Build history of the part. All positions in model axes, mm. Face numbers are marked on the shaded views. A direction names the side the tool comes from. Give positions to 0.01 mm unless a question says otherwise; leave off trailing zeros. Order: outer loops, then holes, each group sorted by start corner. A loop starts at its lowest first (then second) coordinate and runs counter-clockwise, first axis right, second up. Notation, with made-up numbers: (12.5, 2.5) -> (26.5, 2.5) arc R29 ccw to (26.5, 39.5) -> close; hole circle Ø2 at (12, 46.5). An arc over 180 degrees is marked (long way). One line per question, with ' | ' between items. Start each with the question number.
(1) Pull direction Z, two halves, no side cores. Call the marked faces 1, 2, 3 and 4: +Z half, -Z half, draft (parallel to the pull), parting line (faces both ways), or undercut.
(2) Cut at A-A (x = -23.95). Give the cut face in (y, z).
(3) Cut at C-C (y = -3). Give the cut face in (x, z), then the cut area to 3 significant figures.
(4) Cut at B-B (z = 16.5). Give the cut face in (x, y), then the cut area to 3 significant figures.
(5) Cut at D-D (x = -9). Give the cut face in (y, z), then the cut area to 3 significant figures.
(6) Drill centre lines: L1, parallel to Z at x = -22, y = -3.5; L2, parallel to Y at x = -23.95, z = -2; L3, parallel to Z at x = 3, y = 10. Where is each one in solid material? Low to high. Write a range as from..to.
(7) Which spindle directions (+Z, -Z, +X, -X, +Y, -Y) get a long thin tool onto all of the face, cutting with end or side? Do the marked faces 5, 6, 7 and 8. Say none if no direction does.
(8) Pin check, flat tips, straight feed: pin 1 Ø5 at (x, z) = (-8, -15) entering from -Y; pin 2 Ø6 at (x, y) = (-23.95, -9) entering from -Z; pin 3 Ø3 at (x, z) = (-35.5, 3) entering from +Y; pin 4 Ø6 at (x, z) = (13, 16.5) entering from -Y. Stop position of each tip, or through.
from build123d import *
from build123d.topology import SkipClean

# Parameters (mm, degrees)
SKETCH2_W               = 76.3
SKETCH2_H               = 48.2
BOSS_EXTRUDE1_DEPTH     = 4
BOSS_EXTRUDE2_DEPTH     = 15
SKETCH10_W              = 4
SKETCH10_H              = 40.2
BOSS_EXTRUDE5_DEPTH     = 2
CUT_EXTRUDE1_DEPTH      = 3
CUT_EXTRUDE1_DEPTH_BACK = 4
SKETCH5_W               = 13
SKETCH5_H               = 11.2
CUT_EXTRUDE2_REACH      = 66.34
CUT_EXTRUDE3_DEPTH      = 7.5
FILLET3_R               = 1
SKETCH17_W              = 76.3
SKETCH17_H              = 8
SKETCH17_H_2            = 6
BOSS_EXTRUDE6_DEPTH     = 15
SKETCH20_R              = 2.55
CUT_EXTRUDE5_DEPTH      = 65.340209
FILLET4_R               = 1
FILLET5_R               = 1
SKETCH21_W              = 68.3
SKETCH21_H              = 40.2
CUT_EXTRUDE6_DEPTH      = 2
SKETCH29_R              = 2.55
BOSS_EXTRUDE9_DEPTH     = 40.2
SKETCH30_W              = 17.4
SKETCH30_H              = 15
SKETCH30_W_2            = 11.6
SKETCH30_W_3            = 6.4
CUT_EXTRUDE12_DEPTH     = 83.240501


with BuildPart() as part:
    # Sketch2 → Boss-Extrude1 (new body)
    with BuildSketch(Plane(origin=(0, 0, 0), x_dir=(1, 0, 0), z_dir=(0, 1, 0))):
        Rectangle(SKETCH2_W, SKETCH2_H)
    extrude(amount=BOSS_EXTRUDE1_DEPTH)

    # Sketch3 → Boss-Extrude2 (add)
    with BuildSketch(Plane(origin=(0, 4, 0), x_dir=(1, 0, 0), z_dir=(0, 1, 0))):
        Polygon((38.15, 24.1), (-38.15, 24.1), (-38.15, 20.1), (-34.15, 20.1), (34.15, 20.1), (38.15, 20.1), align=None)
        Polygon((-38.15, -24.1), (38.15, -24.1), (38.15, -20.1), (34.15, -20.1), (-34.15, -20.1), (-38.15, -20.1), align=None)
    extrude(amount=BOSS_EXTRUDE2_DEPTH)

    # Sketch10 → Boss-Extrude5 (add)
    with BuildSketch(Plane(origin=(0, 4, 0), x_dir=(1, 0, 0), z_dir=(0, 1, 0))):
        with Locations((-36.15, 0)):
            Rectangle(SKETCH10_W, SKETCH10_H)
        with Locations((36.15, 0)):
            Rectangle(SKETCH10_W, SKETCH10_H)
    extrude(amount=BOSS_EXTRUDE5_DEPTH)

    # Sketch5 → Cut-Extrude1 (cut, two sides: drawn at the far end of the back side and taken through both)
    with BuildSketch(Plane(origin=(0, 4, 0), x_dir=(1, 0, 0), z_dir=(0, 1, 0)).offset(-CUT_EXTRUDE1_DEPTH_BACK)):
        with Locations((12.45, -18.5)):
            Rectangle(SKETCH5_W, SKETCH5_H)
    extrude(amount=CUT_EXTRUDE1_DEPTH + CUT_EXTRUDE1_DEPTH_BACK, mode=Mode.SUBTRACT)

    # Sketch8 → Cut-Extrude2 (cut, up to next)
    with BuildSketch(Plane.XY.offset(24.1), mode=Mode.PRIVATE) as cut_extrude2_sk1:
        with BuildLine():
            Line((2.65, 19), (13.65, 19))
            ThreePointArc((13.65, 19), (14.71066, 18.56066), (15.15, 17.5))
            Line((15.15, 17.5), (15.15, 14.5))
            ThreePointArc((15.15, 14.5), (14.71066, 13.43934), (13.65, 13))
            Line((13.65, 13), (2.65, 13))
            ThreePointArc((2.65, 13), (1.58934, 13.43934), (1.15, 14.5))
            Line((1.15, 14.5), (1.15, 17.5))
            ThreePointArc((1.15, 17.5), (1.58934, 18.56066), (2.65, 19))
        make_face()
    cut_extrude2_tool1 = extrude(cut_extrude2_sk1.sketch, amount=-CUT_EXTRUDE2_REACH, mode=Mode.PRIVATE) & part.part
    add(cut_extrude2_tool1.solids().sort_by_distance((8.15, 16, 24.1))[0], mode=Mode.SUBTRACT)

    # Sketch13 → Cut-Extrude3 (cut, symmetric)
    with BuildSketch(Plane.XY):
        Polygon((38.15, 4), (37.15, 4), (38.15, 2), align=None)
    cut_extrude3 = extrude(amount=CUT_EXTRUDE3_DEPTH, both=True, mode=Mode.SUBTRACT)

    # Mirror2: Cut-Extrude3 across plane
    add(cut_extrude3.mirror(Plane(origin=(0, 0, 0), x_dir=(0, 0, 1), z_dir=(1, 0, 0))), mode=Mode.SUBTRACT)

    # Fillet3
    fillet3_edges = [part.edges().sort_by_distance(p)[0] for p in [
        (0, 0, -24.1),
    ]]
    fillet(fillet3_edges, radius=FILLET3_R)

    # Sketch17 → Boss-Extrude6 (add)
    with BuildSketch(Plane.XZ):
        with Locations((0, 20.1)):
            Rectangle(SKETCH17_W, SKETCH17_H)
        with Locations((0, 6.7)):
            Rectangle(SKETCH17_W, SKETCH17_H_2)
    extrude(amount=BOSS_EXTRUDE6_DEPTH)

    # Sketch20 → Cut-Extrude5 (cut, through all)
    with BuildSketch(Plane.XY.offset(24.1)):
        with Locations((23.95, -9)):
            Circle(SKETCH20_R)
        with Locations((-23.95, -9)):
            Circle(SKETCH20_R)
    extrude(amount=-CUT_EXTRUDE5_DEPTH, mode=Mode.SUBTRACT)

    # Fillet4
    fillet4_edges = [part.edges().sort_by_distance(p)[0] for p in [
        (-38.15, -15, 20.1),
        (38.15, -15, 20.1),
        (-38.15, -15, 6.7),
        (38.15, -15, 6.7),
    ]]
    fillet(fillet4_edges, radius=FILLET4_R)

    # Fillet5
    fillet5_edges = [part.edges().sort_by_distance(p)[0] for p in [
        (1.58934, 18.56066, 24.1),
        (1.15, 16, 24.1),
        (1.58934, 13.43934, 24.1),
        (8.15, 13, 24.1),
        (14.71066, 13.43934, 24.1),
        (15.15, 16, 24.1),
        (14.71066, 18.56066, 24.1),
        (1.15, 16, 20.1),
        (1.58934, 18.56066, 20.1),
        (14.71066, 18.56066, 20.1),
        (15.15, 16, 20.1),
        (14.71066, 13.43934, 20.1),
        (8.15, 13, 20.1),
        (1.58934, 13.43934, 20.1),
        (12.45, 7, 24.1),
        (5.95, 5.5, 20.1),
        (18.95, 5.5, 20.1),
        (5.95, 4, 16.5),
        (18.95, 4, 16.5),
        (12.45, 4, 12.9),
        (12.45, 7, 20.1),
    ]]
    fillet(fillet5_edges, radius=FILLET5_R)

    # Sketch21 → Cut-Extrude6 (cut)
    with BuildSketch(Plane(origin=(0, 4, 0), x_dir=(1, 0, 0), z_dir=(0, 1, 0))):
        Rectangle(SKETCH21_W, SKETCH21_H)
    extrude(amount=-CUT_EXTRUDE6_DEPTH, mode=Mode.SUBTRACT)

    # Sketch29 → Boss-Extrude9 (add, through all)
    with SkipClean():  # the faces are left unmerged after this step: merging them gives an invalid solid
        with BuildSketch(Plane(origin=(0, 0, 16.1), x_dir=(-1, 0, 0), z_dir=(0, 0, -1))):
            with BuildLine():
                Line((-37.15, -15), (37.15, -15))
                ThreePointArc((37.15, -15), (37.857107, -14.707107), (38.15, -14))
                Line((38.15, -14), (38.15, 0))
                Line((38.15, 0), (-5.95, 0))
                Line((-5.95, 0), (-18.95, 0))
                Line((-18.95, 0), (-38.15, 0))
                Line((-38.15, 0), (-38.15, -14))
                ThreePointArc((-38.15, -14), (-37.857107, -14.707107), (-37.15, -15))
            make_face()
            with Locations(Location((-23.95, -9, 0), (0, 0, 180))):
                Circle(SKETCH29_R, mode=Mode.SUBTRACT)
            with Locations((23.95, -9)):
                Circle(SKETCH29_R, mode=Mode.SUBTRACT)
        extrude(amount=BOSS_EXTRUDE9_DEPTH)

    # Sketch30 → Cut-Extrude12 (cut, through all)
    with BuildSketch(Plane(origin=(38.15, 0, 0), x_dir=(0, 0, -1), z_dir=(1, 0, 0))):
        with Locations((15.4, -7.5)):
            Rectangle(SKETCH30_W, SKETCH30_H)
        with Locations((-18.3, -7.5)):
            Rectangle(SKETCH30_W_2, SKETCH30_H)
        with Locations((-2.9, -7.5)):
            Rectangle(SKETCH30_W_3, SKETCH30_H)
    extrude(amount=-CUT_EXTRUDE12_DEPTH, mode=Mode.SUBTRACT)


solid = part.part
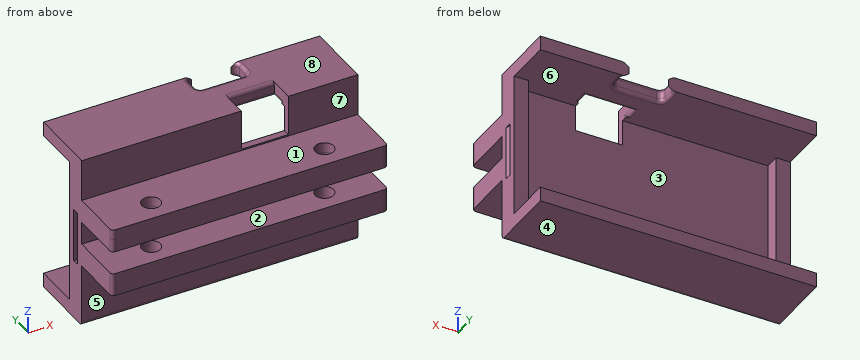
Result set:
1) face 1: +Z half | face 2: undercut | face 3: undercut | face 4: -Z half
2) outline: (-15, -6.7) -> (-11.55, -6.7) -> (-11.55, -0.3) -> (-15, -0.3) -> close; (-15, 6.1) -> (-11.55, 6.1) -> (-11.55, 12.5) -> (-15, 12.5) -> close; (-6.45, -6.7) -> (0, -6.7) -> (0, -23.1) arc R1 ccw to (1, -24.1) -> (19, -24.1) -> (19, -20.1) -> (2, -20.1) -> (2, 20.1) -> (19, 20.1) -> (19, 24.1) -> (0, 24.1) -> (0, 12.5) -> (-6.45, 12.5) -> (-6.45, 6.1) -> (0, 6.1) -> (0, -0.3) -> (-6.45, -0.3) -> close
3) outline: (-38.15, -6.7) -> (38.15, -6.7) -> (38.15, -0.3) -> (-38.15, -0.3) -> close; (-38.15, 6.1) -> (38.15, 6.1) -> (38.15, 12.5) -> (-38.15, 12.5) -> close | area: 977 mm2
4) outline: (-38.15, 0) -> (5.95, 0) -> (5.95, 2) -> (-34.15, 2) -> (-34.15, 6) -> (-38.15, 6) -> close; (18.95, 0) -> (38.15, 0) -> (38.15, 6) -> (34.15, 6) -> (34.15, 2) -> (18.95, 2) -> close | area: 159 mm2
5) outline: (-15, -6.7) -> (0, -6.7) -> (0, -23.1) arc R1 ccw to (1, -24.1) -> (19, -24.1) -> (19, -20.1) -> (2, -20.1) -> (2, 20.1) -> (19, 20.1) -> (19, 24.1) -> (0, 24.1) -> (0, 12.5) -> (-15, 12.5) -> (-15, 6.1) -> (0, 6.1) -> (0, -0.3) -> (-15, -0.3) -> close | area: 424 mm2
6) L1: z = -6.7..-0.3, 6.1..12.5 | L2: y = -15..-11.55, -6.45..2 | L3: z = -24.1..-20.1, 20.1..24.1
7) face 5: -Z, +X, -X, -Y | face 6: +Y | face 7: +Z, +X, -X, -Y | face 8: +Z, +X, -X, +Y, -Y
8) pin 1: stops at y = 0 | pin 2: stops at z = -6.7 | pin 3: stops at y = 6 | pin 4: passes through
